Could you check a few things on this model? Use its own coordinates, in mm. A direction names the side the tool comes from. Give positions to 0.01 mm unless a question says otherwise; leave off trailing zeros. Loops run counter-clockwise (first coordinate to the right, second up) from the corner with the lowest first, then second, coordinate; pieces in that order, holes last. Notation, with made-up numbers: M 62.5,-40 L 119.5,-40 A7 ccw 119.5,-29 Z; hole C 25,-13 d7. An arc over 180 degrees is marked long. Answer in a Markdown table with one row per item. Add a question column.
1. Which directions (+Z, -Z, +X, -X, +Y, -Y) give clear straight access to the entire face, cutting with the end or side of a thin tool? Please do faces 4 (the flat face through (17.326, 9.869, 0.783)), 5 (the cylindrical face through (-13.579, -0.954, 1.565)), 6 (the flat face through (0, 0, 1.588)).
2. If we section it at C-C on y = -10: List the corners of the cut face in (x, z) for me, then the cut area to 3 significant figures.
3. Thinking about a two-plate mould opening in X: for faces 1 (the flat face through (7, 16, 4.762)), 2 (the flat face through (10, 16, 3.175)), 3 (the flat face through (-17.21, 10.07, 0.78)), which applies, released by +X, released by -X, zero draft, split by the parting line, or undercut?
4. If we section it at D-D on x = 3.5: List the corners of the cut face in (y, z) for me, then the cut area to 3 significant figures.
5. I need wall thicknesses on line 1 along Y through (x, z) = (9, 2.5); line 2 along X through (y, z) = (-14.5, 2.5); line 3 along Z through (x, y) = (4, 3). Which ranges of each line are inside material? Lowest first, please. Write a range as from..to.
6. I'm going to push flat-ended pins straight in: pin 1 Ø7 at (x, y) = (-16.5, -0.5) entering from -Z; pin 2 Ø4 at (x, y) = (8.3, -14.38) entering from -Z (3 decimals); pin 3 Ø1.5 at (x, z) = (13.5, 1.5) entering from +Y; pin 4 Ø5 at (x, y) = (-13.5, 13) entering from +Z. Where does each tip first touch, or does it pass through?
7. If we section it at A-A on z = 3.8: List the corners of the cut face in (x, y) for me, then the cut area to 3 significant figures.
8. If we section it at B-B on x = -17: List the corners of the cut face in (y, z) for me (1 decimal), then the cut area to 3 significant figures.
```python
from build123d import *

# Parameters (mm, degrees)
F0_R     = 1.63322
F1_DEPTH = 1.5875
F2_R     = 5.55625
F3_R     = 1.63322
F4_DEPTH = 3.175
F6_R     = 3.175
F7_DEPTH = 3.175


# Not quite as in the source:
# - after a boolean that leaves OpenCascade's solid faulty, fix() repairs it
# - a pattern or mirror of a feature is missing from the dataset's text; its kind, count and spacing are read off the source's solid


with BuildPart() as f1:
    # F0 (on Top) → F1 (new body)
    with BuildSketch(Plane.XY):
        Polygon((11.5116069332, 19.938688085), (-11.5116069332, 19.938688085), (-23.0232138664, 0), (-11.5116069332, -19.938688085), (11.5116069332, -19.938688085), (23.0232138664, 0), align=None)
        with Locations((8.3037045, -14.382438085)):
            Circle(F0_R, mode=Mode.SUBTRACT)
        with Locations((-16.607409, 0)):
            Circle(F0_R, mode=Mode.SUBTRACT)
        with Locations((8.3037045, 14.382438085)):
            Circle(F0_R, mode=Mode.SUBTRACT)
    extrude(amount=F1_DEPTH)

    # F2
    f2_edges = [f1.edges().sort_by_distance(p)[0] for p in [
        (-23.023214, 0, 0.79375),
        (-11.511607, -19.938688, 0.79375),
        (11.511607, -19.938688, 0.79375),
        (23.023214, 0, 0.79375),
        (11.511607, 19.938688, 0.79375),
        (-11.511607, 19.938688, 0.79375),
    ]]
    fillet(f2_edges, radius=F2_R)

    # F3 (on face) → F4 (join)
    with BuildSketch(Plane.XY.offset(1.5875)):
        with BuildLine():
            ThreePointArc((13.1155581498, -17.160563085), (13.6706298723, -15.8205014044), (13.8599545, -14.382438085))
            ThreePointArc((13.8599545, -14.382438085), (4.374842447, -10.4535760321), (8.3037045, -19.938688085))
            ThreePointArc((8.3037045, -19.938688085), (11.0818295, -19.1942917348), (13.1155581498, -17.160563085))
        make_face()
        with Locations((8.3037045, -14.382438085)):
            Circle(F3_R, mode=Mode.SUBTRACT)
        with BuildLine():
            ThreePointArc((-21.4192626498, 2.778125), (-22.163659, 0), (-21.4192626498, -2.778125))
            ThreePointArc((-21.4192626498, -2.778125), (-15.1693456806, -5.3669253723), (-11.051159, 0))
            ThreePointArc((-11.051159, 0), (-15.1693456806, 5.3669253723), (-21.4192626498, 2.778125))
        make_face()
        with Locations((-16.607409, 0)):
            Circle(F3_R, mode=Mode.SUBTRACT)
    f4 = extrude(amount=F4_DEPTH)

    # F4_copies: F4 across plane
    add(f4.mirror(Plane.ZX))

    add(f1.part.fix(), mode=Mode.REPLACE)

    # F6 (on face) → F7 (cut, through all)
    with BuildSketch(Plane(origin=(0, 0, 0), x_dir=(1, 0, 0), z_dir=(0, 0, -1))):
        with Locations((8.3037045, 14.382438085)):
            Circle(F6_R)
        with Locations((8.3037045, -14.382438085)):
            Circle(F6_R)
        with Locations((-16.607409, 0)):
            Circle(F6_R)
    extrude(amount=-F7_DEPTH, mode=Mode.SUBTRACT)


solid = f1.part
```
Results:
| question | item | result |
|---|---|---|
| 1 | face 4 | +Z, -Z, +X, +Y |
| 1 | face 5 | -Z |
| 1 | face 6 | +Z |
| 2 | outline | M -17.25,0 L 17.25,0 L 17.25,1.59 L 11.72,1.59 L 11.72,4.76 L 4.89,4.76 L 4.89,1.59 L -17.25,1.59 Z |
| 2 | area | 76.5 mm2 |
| 3 | face 1 | zero draft |
| 3 | face 2 | undercut |
| 3 | face 3 | released by -X |
| 4 | outline | M -19.94,0 L 19.94,0 L 19.94,1.59 L 17.17,1.59 L 17.17,4.76 L 11.59,4.76 L 11.59,1.59 L -11.59,1.59 L -11.59,4.76 L -17.17,4.76 L -17.17,1.59 L -19.94,1.59 Z |
| 4 | area | 98.8 mm2 |
| 5 | line 1 | -19.89..-17.48, -11.28..-8.87, 8.87..11.28, 17.48..19.89 |
| 5 | line 2 | 2.75..5.13, 11.48..13.86 |
| 5 | line 3 | 0..1.59 |
| 6 | pin 1 | z = 0 |
| 6 | pin 2 | z = 3.175 |
| 6 | pin 3 | y = 17.71 |
| 6 | pin 4 | z = 1.59 |
| 7 | outline | C -16.61,0 d11.11; C 8.3,-14.38 d11.11; C 8.3,14.38 d11.11; hole C -16.61,0 d3.27; hole C 8.3,-14.38 d3.27; hole C 8.3,14.38 d3.27 |
| 7 | area | 266 mm2 |
| 8 | outline | M -10.4,0 L -3.2,0 L -3.2,3.2 L -1.6,3.2 L -1.6,4.8 L -5.5,4.8 L -5.5,1.6 L -10.4,1.6 Z; M 1.6,3.2 L 3.2,3.2 L 3.2,0 L 10.4,0 L 10.4,1.6 L 5.5,1.6 L 5.5,4.8 L 1.6,4.8 Z |
| 8 | area | 43.3 mm2 |
